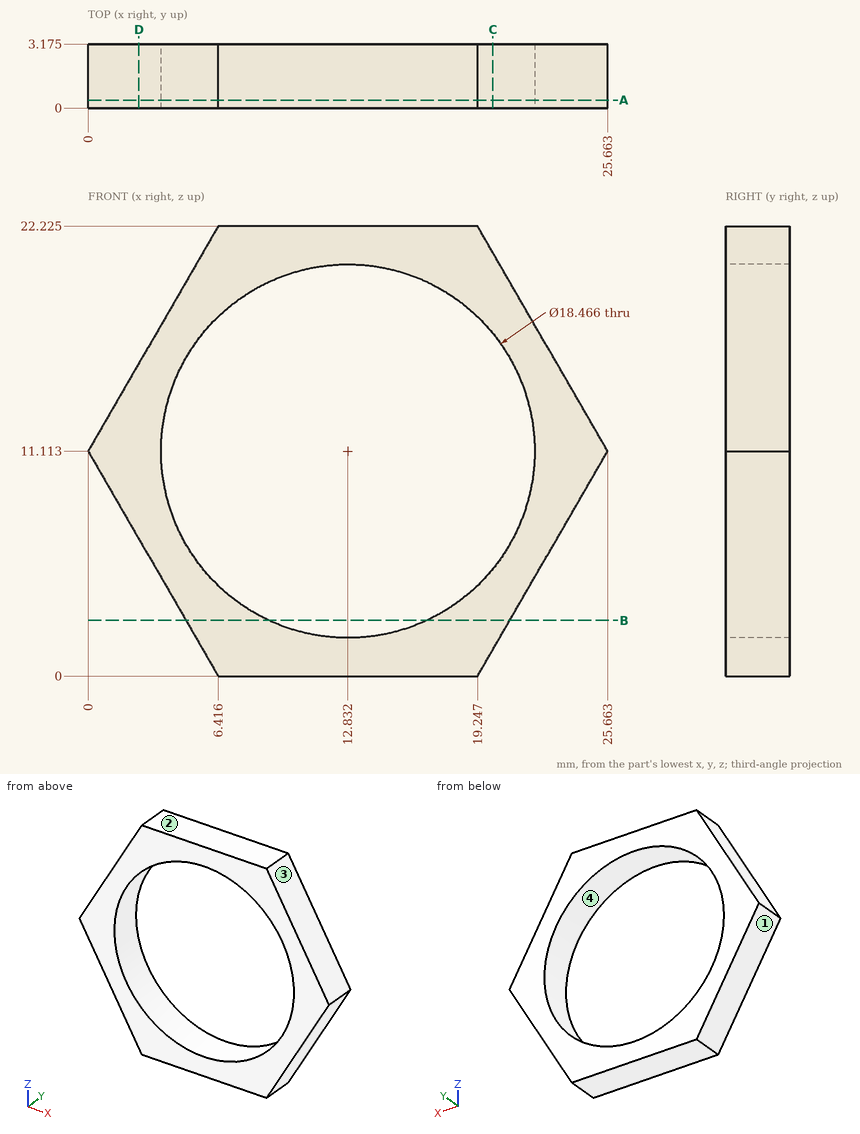
For this review, use the dimensioned drawing (mm, ordinates from the lowest corner) and the shaded views. Round coordinates to 2 decimals unless told otherwise and drop trailing zeros. Order: outer loops, then holes, each group sorted by start corner. A loop starts at its lowest first (then second) coordinate and runs counter-clockwise, first axis right, second up. Notation, with made-up numbers: (76.5, -8) -> (122.5, -8) arc R23 cw to (122.5, 5) -> close; hole circle Ø10 at (22, 74.5). An arc over 180 degrees is marked (long way). Use CSV: the item, a comma, the result in double quotes. Start each with the question number.
(1) Consider section A-A on y = 0.4. Write out the cut boundary in (x, z) (1 decimal).
(2) Consider section C-C on x = 20. Write out the cut boundary in (y, z) (1 decimal).
(3) Consider section B-B on z = 2.75. Write out the cut boundary in (x, y) (1 decimal).
(4) Consider section D-D on x = 2.5. Write out the cut boundary in (y, z) (1 decimal), and give its area (3 significant figures).
(5) Mouldability with a two-part tool opening along X and no side actions: class the marked faces 1, 2, 3 and 4 as pulls with the +X half, pulls with the -X half, needs draft (parallel to the pull), parting line crosses it, or undercut.
(6) Wall thickness on probe 1 along Z at (x, y) = (19.5, 0.85) (1 decimal); probe 2 along X at (y, z) = (3.05, 9) (1 decimal); probe 3 along Z at (x, y) = (9.5, 0.5) (1 decimal): over which ranges is each line inside the solid? List them lowest first. Write a range as from..to.
Responses:
1,outline,"(0, 11.1) -> (6.4, 0) -> (19.2, 0) -> (25.7, 11.1) -> (19.2, 22.2) -> (6.4, 22.2) -> close; hole circle Ø18.5 at (12.8, 11.1)"
2,outline,"(0, 1.3) -> (3.2, 1.3) -> (3.2, 5.3) -> (0, 5.3) -> close; (0, 16.9) -> (3.2, 16.9) -> (3.2, 20.9) -> (0, 20.9) -> close"
3,outline,"(4.8, 0) -> (8.9, 0) -> (8.9, 3.2) -> (4.8, 3.2) -> close; (16.7, 0) -> (20.8, 0) -> (20.8, 3.2) -> (16.7, 3.2) -> close"
4,outline,"(0, 6.8) -> (3.2, 6.8) -> (3.2, 15.4) -> (0, 15.4) -> close"
4,area,"27.5 mm²"
5,face 1,"pulls with the -X half"
5,face 2,"needs draft"
5,face 3,"pulls with the +X half"
5,face 4,"undercut"
6,probe 1,"0.4..4.7, 17.5..21.8"
6,probe 2,"1.2..3.8, 21.8..24.4"
6,probe 3,"0..2.5, 19.7..22.2"
